from build123d import *

# Parameters (mm, degrees)
BOSS_EXTRUDE5_START = 4.25
BOSS_EXTRUDE5_DEPTH = 6
CUT_EXTRUDE2_DEPTH  = 92.979276087
SKETCH4_R           = 1.575
CUT_EXTRUDE3_DEPTH  = 10


with BuildPart() as part:
    # Sketch2 → Boss-Extrude5 (new body)
    with BuildSketch(Plane.XY.offset(BOSS_EXTRUDE5_START)):
        with BuildLine():
            ThreePointArc((68.209851787, 17.593254842), (67.854853617, 17.589672886), (67.5, 17.578928476))
            ThreePointArc((67.5, 17.578928476), (61.469163108, 16.250714817), (56.268821721, 12.920310248))
            ThreePointArc((56.268821721, 12.920310248), (61.039234507, 7.227490774), (62.750493933, 0))
            Line((62.750493933, 0), (65.559851787, 0))
            ThreePointArc((65.559851787, 0), (66.336018817, 1.87383297), (68.209851787, 2.65))
            Line((68.209851787, 2.65), (68.209851787, 17.593254842))
        make_face()
        with BuildLine():
            ThreePointArc((56.268821721, -12.920310248), (61.469163108, -16.250714817), (67.5, -17.578928476))
            ThreePointArc((67.5, -17.578928476), (67.854853617, -17.589672886), (68.209851787, -17.593254842))
            Line((68.209851787, -17.593254842), (68.209851787, -2.65))
            ThreePointArc((68.209851787, -2.65), (66.336018817, -1.87383297), (65.559851787, 0))
            Line((65.559851787, 0), (62.750493933, 0))
            ThreePointArc((62.750493933, 0), (61.039234507, -7.227490774), (56.268821721, -12.920310248))
        make_face()
        with BuildLine():
            ThreePointArc((62.750493933, 0), (61.039234507, 7.227490774), (56.268821721, 12.920310248))
            ThreePointArc((56.268821721, 12.920310248), (52.091474062, 7.051277576), (50.616596945, 0))
            Line((50.616596945, 0), (62.750493933, 0))
        make_face()
        with BuildLine():
            ThreePointArc((50.616596945, 0), (52.091474062, -7.051277576), (56.268821721, -12.920310248))
            ThreePointArc((56.268821721, -12.920310248), (61.039234507, -7.227490774), (62.750493933, 0))
            Line((62.750493933, 0), (50.616596945, 0))
        make_face()
        with BuildLine():
            ThreePointArc((62.750493933, 0), (61.039234507, 7.227490774), (56.268821721, 12.920310248))
            ThreePointArc((56.268821721, 12.920310248), (52.091474062, 7.051277576), (50.616596945, 0))
            Line((50.616596945, 0), (62.750493933, 0))
        make_face()
        with BuildLine():
            ThreePointArc((50.616596945, 0), (52.091474062, -7.051277576), (56.268821721, -12.920310248))
            ThreePointArc((56.268821721, -12.920310248), (61.039234507, -7.227490774), (62.750493933, 0))
            Line((62.750493933, 0), (50.616596945, 0))
        make_face()
        with BuildLine():
            ThreePointArc((68.209851787, 17.593254842), (67.854853617, 17.589672886), (67.5, 17.578928476))
            ThreePointArc((67.5, 17.578928476), (61.469163108, 16.250714817), (56.268821721, 12.920310248))
            ThreePointArc((56.268821721, 12.920310248), (61.039234507, 7.227490774), (62.750493933, 0))
            Line((62.750493933, 0), (65.559851787, 0))
            ThreePointArc((65.559851787, 0), (66.336018817, 1.87383297), (68.209851787, 2.65))
            Line((68.209851787, 2.65), (68.209851787, 17.593254842))
        make_face()
        with BuildLine():
            ThreePointArc((56.268821721, -12.920310248), (61.469163108, -16.250714817), (67.5, -17.578928476))
            ThreePointArc((67.5, -17.578928476), (67.854853617, -17.589672886), (68.209851787, -17.593254842))
            Line((68.209851787, -17.593254842), (68.209851787, -2.65))
            ThreePointArc((68.209851787, -2.65), (66.336018817, -1.87383297), (65.559851787, 0))
            Line((65.559851787, 0), (62.750493933, 0))
            ThreePointArc((62.750493933, 0), (61.039234507, -7.227490774), (56.268821721, -12.920310248))
        make_face()
        with BuildLine():
            ThreePointArc((78.767770494, 14.073129307), (73.774493088, 16.69003844), (68.209851787, 17.593254842))
            Line((68.209851787, 17.593254842), (68.209851787, 2.65))
            ThreePointArc((68.209851787, 2.65), (70.083684757, 1.87383297), (70.859851787, 0))
            Line((70.859851787, 0), (71.993520086, 0))
            ThreePointArc((71.993520086, 0), (73.775238341, 7.809344356), (78.767770494, 14.073129307))
        make_face()
        with BuildLine():
            Line((68.209851787, -2.65), (68.209851787, -17.593254842))
            ThreePointArc((68.209851787, -17.593254842), (73.774493088, -16.69003844), (78.767770494, -14.073129307))
            ThreePointArc((78.767770494, -14.073129307), (73.775238341, -7.809344356), (71.993520086, 0))
            Line((71.993520086, 0), (70.859851787, 0))
            ThreePointArc((70.859851787, 0), (70.083684757, -1.87383297), (68.209851787, -2.65))
        make_face()
        with BuildLine():
            ThreePointArc((78.767770494, 14.073129307), (73.774493088, 16.69003844), (68.209851787, 17.593254842))
            Line((68.209851787, 17.593254842), (68.209851787, 2.65))
            ThreePointArc((68.209851787, 2.65), (70.083684757, 1.87383297), (70.859851787, 0))
            Line((70.859851787, 0), (71.993520086, 0))
            ThreePointArc((71.993520086, 0), (73.775238341, 7.809344356), (78.767770494, 14.073129307))
        make_face()
        with BuildLine():
            Line((68.209851787, -2.65), (68.209851787, -17.593254842))
            ThreePointArc((68.209851787, -17.593254842), (73.774493088, -16.69003844), (78.767770494, -14.073129307))
            ThreePointArc((78.767770494, -14.073129307), (73.775238341, -7.809344356), (71.993520086, 0))
            Line((71.993520086, 0), (70.859851787, 0))
            ThreePointArc((70.859851787, 0), (70.083684757, -1.87383297), (68.209851787, -2.65))
        make_face()
        with BuildLine():
            add(Edge.make_bspline(
                [(90, 18.005197753), (87.300427685, 18.005389985), (81.17457593, 17.968478919), (73.674128402, 17.806885767), (68.874876564, 17.634447138), (67.5, 17.578928476)],
                knots=[0.344744853, 0.344744853, 0.344744853, 0.344744853, 0.357984483, 0.374788114, 0.381536428, 0.381536428, 0.381536428, 0.381536428], degree=3))
            ThreePointArc((67.5, 17.578928476), (67.854853617, 17.589672886), (68.209851787, 17.593254842))
            ThreePointArc((68.209851787, 17.593254842), (73.774493088, 16.69003844), (78.767770494, 14.073129307))
            ThreePointArc((78.767770494, 14.073129307), (84.049630886, 16.993984573), (90, 18.005197753))
        make_face()
        with BuildLine():
            ThreePointArc((68.209851787, -17.593254842), (67.854853617, -17.589672886), (67.5, -17.578928476))
            add(Edge.make_bspline(
                [(67.5, -17.578928476), (68.874876564, -17.634447138), (73.674128402, -17.806885767), (81.17457593, -17.968478919), (87.300427685, -18.005389985), (90, -18.005197753)],
                knots=[0.618463572, 0.618463572, 0.618463572, 0.618463572, 0.625211886, 0.642015517, 0.655255147, 0.655255147, 0.655255147, 0.655255147], degree=3))
            ThreePointArc((90, -18.005197753), (84.049630886, -16.993984573), (78.767770494, -14.073129307))
            ThreePointArc((78.767770494, -14.073129307), (73.774493088, -16.69003844), (68.209851787, -17.593254842))
        make_face()
        with BuildLine():
            add(Edge.make_bspline(
                [(90, 18.005197753), (87.300427685, 18.005389985), (81.17457593, 17.968478919), (73.674128402, 17.806885767), (68.874876564, 17.634447138), (67.5, 17.578928476)],
                knots=[0.344744853, 0.344744853, 0.344744853, 0.344744853, 0.357984483, 0.374788114, 0.381536428, 0.381536428, 0.381536428, 0.381536428], degree=3))
            ThreePointArc((67.5, 17.578928476), (67.854853617, 17.589672886), (68.209851787, 17.593254842))
            ThreePointArc((68.209851787, 17.593254842), (73.774493088, 16.69003844), (78.767770494, 14.073129307))
            ThreePointArc((78.767770494, 14.073129307), (84.049630886, 16.993984573), (90, 18.005197753))
        make_face()
        with BuildLine():
            ThreePointArc((68.209851787, -17.593254842), (67.854853617, -17.589672886), (67.5, -17.578928476))
            add(Edge.make_bspline(
                [(67.5, -17.578928476), (68.874876564, -17.634447138), (73.674128402, -17.806885767), (81.17457593, -17.968478919), (87.300427685, -18.005389985), (90, -18.005197753)],
                knots=[0.618463572, 0.618463572, 0.618463572, 0.618463572, 0.625211886, 0.642015517, 0.655255147, 0.655255147, 0.655255147, 0.655255147], degree=3))
            ThreePointArc((90, -18.005197753), (84.049630886, -16.993984573), (78.767770494, -14.073129307))
            ThreePointArc((78.767770494, -14.073129307), (73.774493088, -16.69003844), (68.209851787, -17.593254842))
        make_face()
    extrude(amount=BOSS_EXTRUDE5_DEPTH)

    # Sketch3 → Cut-Extrude2 (cut, through all)
    with BuildSketch(Plane.XY.offset(10.25)):
        with BuildLine():
            ThreePointArc((67.512104385, -17.279172769), (50.916596945, 0), (67.512104385, 17.279172769))
            Line((67.512104385, 17.279172769), (69.466542011, 17.654214769))
            add(Edge.make_bspline(
                [(69.466542011, 17.654214769), (68.810976965, 17.630475848), (68.155460296, 17.605396509), (67.5, 17.578928476)],
                knots=[0.378319229, 0.378319229, 0.378319229, 0.378319229, 0.381536428, 0.381536428, 0.381536428, 0.381536428], degree=3))
            ThreePointArc((67.5, 17.578928476), (50.616596945, 0), (67.5, -17.578928476))
            add(Edge.make_bspline(
                [(67.5, -17.578928476), (68.155460296, -17.605396509), (68.810976965, -17.630475848), (69.466542011, -17.654214769)],
                knots=[0.618463572, 0.618463572, 0.618463572, 0.618463572, 0.621680771, 0.621680771, 0.621680771, 0.621680771], degree=3))
            Line((69.466542011, -17.654214769), (67.512104385, -17.279172769))
        make_face()
        with BuildLine():
            add(Edge.make_bspline(
                [(90, 18.005197753), (88.88435893, 18.005277196), (87.768717531, 18.00254573), (86.653091523, 17.996862246)],
                knots=[0.344744853, 0.344744853, 0.344744853, 0.344744853, 0.35021634, 0.35021634, 0.35021634, 0.35021634], degree=3))
            ThreePointArc((86.653091523, 17.996862246), (71.693520086, 0), (86.653091523, -17.996862246))
            add(Edge.make_bspline(
                [(86.653091523, -17.996862246), (87.768717531, -18.00254573), (88.88435893, -18.005277196), (90, -18.005197753)],
                knots=[0.64978366, 0.64978366, 0.64978366, 0.64978366, 0.655255147, 0.655255147, 0.655255147, 0.655255147], degree=3))
            ThreePointArc((90, -18.005197753), (71.993520086, 0), (90, 18.005197753))
        make_face()
    extrude(amount=-CUT_EXTRUDE2_DEPTH, mode=Mode.SUBTRACT)

    # Sketch4 → Cut-Extrude3 (cut)
    with BuildSketch(Plane.XY.offset(10.25)):
        with Locations((65.559851787, 5.4)):
            Circle(SKETCH4_R)
        with Locations((65.559851787, -5.4)):
            Circle(SKETCH4_R)
    extrude(amount=-CUT_EXTRUDE3_DEPTH, mode=Mode.SUBTRACT)


solid = part.part
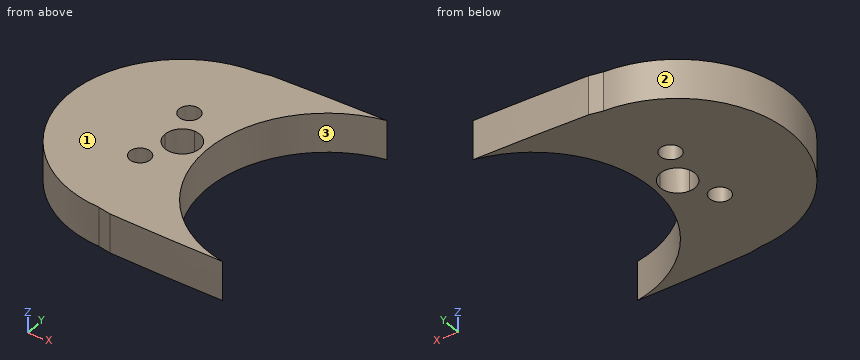
Model file for the job. Use its own axes, mm. Face numbers are marked on the shaded views. Give positions to 0.01 mm unless a question says otherwise; leave off trailing zeros. Loops run counter-clockwise (first coordinate to the right, second up) from the corner with the lowest first, then second, coordinate; pieces in that order, holes last.
Item 1: Slice it at B-B (y = 5.4). Write the cut outline in (x, z), plus the area to 3 significant figures.
Check values:
outline: (51.78, 4.25) - (63.98, 4.25) - (63.98, 10.25) - (51.78, 10.25) - close; (67.13, 4.25) - (72.51, 4.25) - (72.51, 10.25) - (67.13, 10.25) - close
area: 105 mm2
Item 2: Slice it at A-A (x = 65). Write the cut outline in (y, z), plus the area to 3 significant figures.
Check values:
outline: (-16.99, 4.25) - (-6.87, 4.25) - (-6.87, 10.25) - (-16.99, 10.25) - close; (-3.93, 4.25) - (3.93, 4.25) - (3.93, 10.25) - (-3.93, 10.25) - close; (6.87, 4.25) - (16.99, 4.25) - (16.99, 10.25) - (6.87, 10.25) - close
area: 169 mm2
Item 3: Drill centre lines: line 1 along Y through (x, z) = (65, 6.25); line 2 along X through (y, z) = (-6.5, 8); line 3 along Y through (x, z) = (74, 9.5). Where is each one in solid material? Low to high.
Check values:
line 1: y = -16.99 to -6.87, -3.93 to 3.93, 6.87 to 16.99
line 2: x = 52.18 to 64.43, 66.69 to 72.89
line 3: y = -17.8 to -8.9, 8.9 to 17.8
Item 4: Drop a flat-ended pin along its axis: P1, Ø1, axis at y = -12.5, z = 6.5, coming from the -X side. Give the stop position or say it passes through.
Check values:
P1: stops at x = 55.76
Item 5: Slice it at C-C (z = 8.25). Give the number of separate pieces and of enclosed holes in the cut face, plus the area to 3 significant figures.
Check values:
separate pieces: 1
enclosed holes: 3
area: 686 mm2
Item 6: Slice it at D-D (y = -2). Write the cut outline in (x, z).
Check values:
outline: (51.03, 4.25) - (66.47, 4.25) - (66.47, 10.25) - (51.03, 10.25) - close; (69.95, 4.25) - (71.8, 4.25) - (71.8, 10.25) - (69.95, 10.25) - close
Item 7: Mould opens along Y. For the marked faces 1, 2 and 3 say: +Y half, -Y half, draft (parallel to the pull), parting line (faces both ways), or undercut.
Check values:
face 1: draft
face 2: parting line
face 3: undercut
